Geometry: final body of the model. Coordinates: model frame, mm. A direction names the side the tool comes from. Round coordinates to 2 decimals unless told otherwise and drop trailing zeros. Loops run counter-clockwise (first coordinate to the right, second up) from the corner with the lowest first, then second, coordinate; pieces in that order, holes last. Notation, with made-up numbers: (-10.75, 1) - (31.25, 1) arc R17 ccw to (31.25, 15) - close; hole circle Ø6 at (-10, 71). An arc over 180 degrees is marked (long way). Return JSON: item names as keys, results as strings. Group by question number.
1. Section B-B on x = 3.5. Return loops of the section in (y, z), and give its area (3 significant figures).
2. First-contact query: pin 1 Ø0.9 at (y, z) = (-4.5, 1) entering from +X; pin 2 Ø1 at (x, y) = (3, -4.5) entering from -Z. Flat tips, straight axial feed; report the tip coordinate or a pass-through.
3. Material intervals for probe 1 along Z at (x, y) = (4, -5); probe 2 along X at (y, z) = (-1.25, 1.25); probe 3 along X at (y, z) = (-1, 8.75), sorted ascending.
4. Set-up query: faces 1 (the face through (7.22, -2.73, 4.74)), 2 (the face through (-3.501, -4, 5)), 3 (the face through (1.499, -4, 1)). Return all of +Z, -Z, +X, -X, +Y, -Y with unobstructed straight access to the full face (end or side cutting, diameter ignored); none if empty.
5. Section A-A on z = 0.5. Return loops of the section in (x, y), and give its area (3 significant figures).
from build123d import *

# Parameters (mm, degrees)
F1_DEPTH = 8
F2_R     = 2.75
F3_DEPTH = 6
F4_R     = 1.5
F5_R     = 3
F6_R     = 0.5


with BuildPart() as f1:
    # F0 (on Front) → F1 (new body)
    with BuildSketch(Plane.XZ):
        with BuildLine():
            Line((4.9994771853, 12.180397345), (-3.5005228147, 12.180397345))
            Line((-3.5005228147, 12.180397345), (-3.5005228147, -2.819602655))
            Line((-3.5005228147, -2.819602655), (-0.5005228147, -2.819602655))
            ThreePointArc((-0.5005228147, -2.819602655), (0.9136907477, -2.2338162174), (1.4994771853, -0.819602655))
            Line((1.4994771853, -0.819602655), (1.4994771853, 2.180397345))
            Line((1.4994771853, 2.180397345), (4.9994771853, 2.180397345))
            Line((4.9994771853, 2.180397345), (4.9994771853, 12.180397345))
        make_face()
    extrude(amount=F1_DEPTH)

    # F2 (on face) → F3 (join)
    with BuildSketch(Plane.YZ.offset(4.9994771853)):
        with Locations((-4, 7.180397345)):
            Circle(F2_R)
    extrude(amount=F3_DEPTH)

    # F4
    f4_edges = [f1.edges().sort_by_distance(p)[0] for p in [
        (10.999477, -6.75, 7.180397),
    ]]
    fillet(f4_edges, radius=F4_R)

    # F5
    f5_edges = [f1.edges().sort_by_distance(p)[0] for p in [
        (0.749477, 0, 12.180397),
        (0.749477, -8, 12.180397),
    ]]
    fillet(f5_edges, radius=F5_R)

    # F6
    f6_edges = [f1.edges().sort_by_distance(p)[0] for p in [
        (4.999477, -8, 5.680397),
        (4.999477, -7.12132, 11.301718),
        (4.999477, -4, 12.180397),
        (4.999477, -0.87868, 11.301718),
        (4.999477, 0, 5.680397),
        (-3.500523, -8, 3.180397),
        (-3.500523, -7.12132, 11.301718),
    ]]
    fillet(f6_edges, radius=F6_R)


solid = f1.part
Taken from the geometry:
{
 "1": {"outline": "(-8, 2.18) - (0, 2.18) - (0, 9.18) arc R3 ccw to (-3, 12.18) - (-5, 12.18) arc R3 ccw to (-8, 9.18) - close", "area": "76.1 mm2"},
 "2": {"pin 1": "x = 1.5", "pin 2": "z = 2.18"},
 "3": {"probe 1": "2.18 to 12.18", "probe 2": "-3.5 to 1.5", "probe 3": "-3.5 to 5"},
 "4": {"face 1": "+X", "face 2": "+Z, -Z, -X, +Y, -Y", "face 3": "-Z, +X, +Y, -Y"},
 "5": {"outline": "(-3.5, -7.5) arc R0.5 ccw to (-3, -8) - (1.5, -8) - (1.5, 0) - (-3, 0) arc R0.5 ccw to (-3.5, -0.5) - close", "area": "39.9 mm2"}
}
